Autodesk Inventor part; units mm, degrees
ref_plane "YZ Plane" through (0, 0, 0) normal (1, 0, 0) x (0, 1, 0)
ref_plane "XZ Plane" through (0, 0, 0) normal (0, 1, 0) x (-1, 0, 0)
ref_plane "XY Plane" through (0, 0, 0) normal (0, 0, 1) x (1, 0, 0)
ref_plane "Work Plane4" through (0, 0, 0) normal (0, 0, 1) x (1, 0, 0)
sketch "Sketch1" plane through (0, 0, 0) normal (0, 0, 1) x (1, 0, 0)
  line L0 (37, 49) -> (37, -49)
  arc A0 (37, 49) -> (35, 51) centre (35, 49) ccw
  line L1 (-35, 51) -> (35, 51)
  line L2 (-37, -49) -> (-37, 49)
  arc A1 (-35, 51) -> (-37, 49) centre (-35, 49) ccw
  arc A2 (-37, -49) -> (-35, -51) centre (-35, -49) ccw
  line L3 (35, -51) -> (-35, -51)
  arc A3 (35, -51) -> (37, -49) centre (35, -49) ccw
  arc A4 (36.8, 49) -> (35, 50.8) centre (35, 49) ccw
  line L4 (36.8, 49) -> (36.8, -49)
  arc A5 (35, -50.8) -> (36.8, -49) centre (35, -49) ccw
  line L5 (35, -50.8) -> (-35, -50.8)
  arc A6 (-36.8, -49) -> (-35, -50.8) centre (-35, -49) ccw
  line L6 (-36.8, -49) -> (-36.8, 49)
  arc A7 (-35, 50.8) -> (-36.8, 49) centre (-35, 49) ccw
  line L7 (-35, 50.8) -> (35, 50.8)
  point P0 (0, 0)
  point P1 (34.3, 48.3)
  point P2 (-33, 42)
  dimension "d0" = 0.2
extrude "Extrusion1" add sketch "Sketch1" against normal blind 2 contours L4 A5 L5 A6 L6 A7 L7 A4
sketch "Sketch4" plane through (0, 0, 0) normal (0, 0, 1) x (1, 0, 0)
  line L0 (36.8, -49) -> (36.8, 49)
  arc A0 (36.8, 49) -> (35, 50.8) centre (35, 49) ccw
  line L1 (35, 50.8) -> (-35, 50.8)
  arc A1 (-35, 50.8) -> (-36.8, 49) centre (-35, 49) ccw
  line L2 (-36.8, 49) -> (-36.8, -49)
  arc A2 (-36.8, -49) -> (-35, -50.8) centre (-35, -49) ccw
  line L3 (-35, -50.8) -> (35, -50.8)
  arc A3 (35, -50.8) -> (36.8, -49) centre (35, -49) ccw
  circle A4 centre (34.3, 48.3) radius 1.4
  circle A5 centre (34.3, -48.3) radius 1.4
  circle A6 centre (-34.3, -48.3) radius 1.4
  circle A7 centre (-34.3, 48.3) radius 1.4
  point P0 (0, 0)
  dimension "d22" = 2.8
  dimension "d23" = 2.8
  dimension "d24" = 2.8
  dimension "d25" = 2.8
  dimension "d59" = 2.5
  dimension "d60" = 2.5
  dimension "d62" = 2.5
  dimension "d63" = 2.5
  dimension "d64" = 2.5
  dimension "d65" = 2.5
  dimension "d66" = 2.5
  dimension "d67" = 2.5
extrude "Extrusion3" cut sketch "Sketch4" against normal blind 10 contours A4 | A5 | A6 | A7
ref_plane "Work Plane5" through (0, 0, -2) normal (0, 0, -1) x (-1, 0, 0)
sketch "Sketch5" plane through (0, 0, -2) normal (0, 0, -1) x (-1, 0, 0)
  line L0 (-34.8, 48.8) -> (34.8, 48.8)
  line L1 (34.8, 48.8) -> (34.8, -48.8)
  line L2 (34.8, -48.8) -> (-34.8, -48.8)
  line L3 (-34.8, -48.8) -> (-34.8, 48.8)
  circle A0 centre (34.3, 48.3) radius 1.4
  circle A1 centre (34.3, -48.3) radius 1.4
  circle A2 centre (-34.3, -48.3) radius 1.4
  circle A3 centre (-34.3, 48.3) radius 1.4
  circle A4 centre (-34.3, 48.3) radius 2.9
  circle A5 centre (-34.3, -48.3) radius 2.9
  circle A6 centre (34.3, -48.3) radius 2.9
  circle A7 centre (34.3, 48.3) radius 2.9
  circle A8 centre (34.3, -48.3) radius 1.4
  circle A9 centre (34.3, 48.3) radius 1.4
  circle A10 centre (-34.3, -48.3) radius 1.4
  circle A11 centre (-34.3, 48.3) radius 1.4
  line L4 (-36.8, 49) -> (-36.8, -49)
  arc A12 (-36.8, -49) -> (-35, -50.8) centre (-35, -49) ccw
  line L5 (-35, -50.8) -> (35, -50.8)
  arc A13 (35, -50.8) -> (36.8, -49) centre (35, -49) ccw
  line L6 (36.8, -49) -> (36.8, 49)
  arc A14 (36.8, 49) -> (35, 50.8) centre (35, 49) ccw
  line L7 (35, 50.8) -> (-35, 50.8)
  arc A15 (-35, 50.8) -> (-36.8, 49) centre (-35, 49) ccw
  point P0 (0, 0)
  point P1 (-31.4434, 48.8)
  point P2 (31.4434, 48.8)
  point P3 (34.8, 45.4434)
  point P4 (34.8, -45.4434)
  point P5 (31.4434, -48.8)
  point P6 (-31.4434, -48.8)
  point P7 (-34.8, -45.4434)
  point P8 (-34.8, 45.4434)
  dimension "d68" = 1.5
  dimension "d69" = 1.5
  dimension "d70" = 1.5
  dimension "d71" = 1.5
extrude "Extrusion4" add sketch "Sketch5" along normal blind 10.7 contours L3 A3 L0 | L0 A3 L3 | A3 L3 A4 L4 A15 L7 L0 | L0 A4 L3 A3 | A4 L7 A7 L0 | L3 A5 L4 A4 | A7 L7 A14 L6 L1 A0 L0 | L0 A0 L1 A7 | A5 L2 A2 L3 | L3 A2 L2 A5 L5 A12 L4 | A0 L1 L0 | L0 L1 A0 | A7 L6 A6 L1 | A2 L2 L3 | L3 L2 A2 | A6 L6 A13 L5 L2 A1 L1 | L1 A1 L2 A6 | L2 A6 L5 A5 | A1 L2 L1 | L1 L2 A1
sketch "Sketch6" plane through (-34.3, 48.3, -2) normal (0, 0, 1) x (1, 0, 0)
  circle A0 centre (68.6, 0) radius 1.4
  circle A1 centre (0, 0) radius 1.4
  circle A2 centre (0, -96.6) radius 1.4
  circle A3 centre (68.6, -96.6) radius 1.4
  circle A4 centre (68.6, 0) radius 0.8
  circle A5 centre (0, 0) radius 0.8
  circle A6 centre (0, -96.6) radius 0.8
  circle A7 centre (68.6, -96.6) radius 0.8
  point P0 (34.3, -48.3)
  dimension "d47" = 1.6
  dimension "d48" = 1.6
  dimension "d49" = 1.6
  dimension "d50" = 1.6
extrude "Extrusion5" cut sketch "Sketch6" against normal through all contours A4 | A5 | A6 | A7
sketch "Sketch7" plane through (-34.3, 48.3, -2) normal (0, 0, 1) x (1, 0, 0)
  circle A0 centre (0, 0) radius 1.4
  circle A1 centre (0, -96.6) radius 1.4
  circle A2 centre (68.6, -96.6) radius 1.4
  circle A3 centre (68.6, 0) radius 1.4
  point P0 (34.3, -48.3)
extrude "Extrusion6" cut sketch "Sketch7" against normal blind 7.9
sketch "Sketch8" plane through (0, 0, -12.7) normal (0, 0, -1) x (-1, 0, 0)
  circle A0 centre (-34.3, -48.3) radius 0.8
  circle A1 centre (-34.3, 48.3) radius 0.8
  circle A2 centre (34.3, -48.3) radius 0.8
  circle A3 centre (34.3, 48.3) radius 0.8
  arc A4 (-36.8, -49) -> (-35, -50.8) centre (-35, -49) ccw
  line L0 (-35, -50.8) -> (35, -50.8)
  arc A5 (35, -50.8) -> (36.8, -49) centre (35, -49) ccw
  line L1 (36.8, -49) -> (36.8, 49)
  arc A6 (36.8, 49) -> (35, 50.8) centre (35, 49) ccw
  line L2 (35, 50.8) -> (-35, 50.8)
  arc A7 (-35, 50.8) -> (-36.8, 49) centre (-35, 49) ccw
  line L3 (-36.8, 49) -> (-36.8, -49)
  line L4 (-31.4434, 48.8) -> (31.4434, 48.8)
  arc A8 (31.4434, 48.8) -> (34.8, 45.4434) centre (34.3, 48.3) ccw
  line L5 (34.8, 45.4434) -> (34.8, -45.4434)
  arc A9 (34.8, -45.4434) -> (31.4434, -48.8) centre (34.3, -48.3) ccw
  line L6 (31.4434, -48.8) -> (-31.4434, -48.8)
  arc A10 (-31.4434, -48.8) -> (-34.8, -45.4434) centre (-34.3, -48.3) ccw
  line L7 (-34.8, -45.4434) -> (-34.8, 45.4434)
  arc A11 (-34.8, 45.4434) -> (-31.4434, 48.8) centre (-34.3, 48.3) ccw
  line L8 (34.8, 45.4434) -> (34.8, -45.4434)
  line L9 (36.8, 10.8) -> (34.8, 10.8)
  line L10 (34.8, 10.8) -> (34.8, -10.8)
  line L11 (34.8, -10.8) -> (36.8, -10.8)
  line L12 (36.8, -10.8) -> (36.8, 10.8)
  line L13 (35, 50.8) -> (-35, 50.8)
  line L14 (-31.4434, 48.8) -> (31.4434, 48.8)
  line L15 (-6.8, 50.8) -> (6.8, 50.8)
  line L16 (6.8, 50.8) -> (6.8, 48.8)
  line L17 (6.8, 48.8) -> (-6.8, 48.8)
  line L18 (-6.8, 48.8) -> (-6.8, 50.8)
  point P0 (0, 0)
  dimension "d74" = 40
  dimension "d75" = 40
  dimension "d76" = 30
  dimension "d77" = 30
extrude "Extrusion7" cut sketch "Sketch8" against normal blind 8 contours L2 L16 L4 L18 | L11 L5 L9 L1
fillet "Fillet3" radius 2 4 edges at (-35.8, -10.8, -4.7) (-35.8, 10.8, -4.7) (-6.8, 49.8, -4.7) (6.8, 49.8, -4.7)
properties part number "Bottom_lid_3DPrint"
Here's how the part is built. I have some questions about the finished solid (model axes, mm). A direction names the side the tool comes from. Coordinates: 2 decimals unless noted, no trailing zeros. Order: outer loops, then holes, each group sorted by start corner. A loop starts at its lowest first (then second) coordinate and runs counter-clockwise, first axis right, second up.
Item 1: For faces 4 (the face through (35, 49, -9.9)), 5 (the face through (34.8, -1, -7)), 6 (the face through (-36, -10.8, -10)), which set-ups out of +Z, -Z, +X, -X, +Y, -Y let a thin tool reach every point of the face, with its end or its side?
Result sheet:
face 4: +Z
face 5: -Z
face 6: -Z, -X
Item 2: For P1, Ø2.5, axis at x = 34.3, y = 48.3, coming from the +Z side; P2, Ø1.5, axis at x = -29, y = -36.5, coming from the -Z side; P3, Ø1.6, axis at x = -36, z = -10.5, coming from the +Y side, each with a flat end and sliding along its axis, tell me the tip position at first contact or that it passes through.
Result sheet:
P1: stops at z = -9.9
P2: stops at z = -2
P3: stops at y = 50.79
Item 3: If we section it at B-B on y = -19: List the corners of the cut face in (x, z) for me.
Result sheet:
outline: (-36.8, -12.7) - (-34.8, -12.7) - (-34.8, -2) - (34.8, -2) - (34.8, -12.7) - (36.8, -12.7) - (36.8, 0) - (-36.8, 0) - close
Item 4: If we section it at A-A on x = 13: List the corners of the cut face in (y, z) for me, plus the area to 3 significant figures.
Result sheet:
outline: (-50.8, -12.7) - (-48.8, -12.7) - (-48.8, -2) - (48.8, -2) - (48.8, -12.7) - (50.8, -12.7) - (50.8, 0) - (-50.8, 0) - close
area: 246 mm2
Item 5: If we mould it in two halves opening along X, with no side actions, what happens to faces 1 (the face through (-35.41, -49.15, -4.88)), 2 (the face through (-35, 38, -12.7)), 3 (the face through (-36.8, -1, -3))? For each: +X half, -X half, draft (parallel to the pull), parting line (faces both ways), or undercut.
Result sheet:
face 1: undercut
face 2: draft
face 3: -X half
Item 6: I need wall thicknesses on line 1 (Y direction, x = 34.3, z = -6.5); line 2 (Y direction, x = 34.3, z = -10.5); line 3 (X direction, y = 48.3, z = -11.45). Which ranges of each line are inside material? Lowest first, please.
Result sheet:
line 1: y = -50.8 to -49.7, -46.9 to -45.4, 45.4 to 46.9, 49.7 to 50.8
line 2: y = -50.8 to -49.1, -47.5 to -45.4, 45.4 to 47.5, 49.1 to 50.8
line 3: x = -36.8 to -35.1, -33.5 to -31.4, 31.4 to 33.5, 35.1 to 36.8
